Geometry: final body of the model. Coordinates: model frame, mm. A direction names the side the tool comes from. Round coordinates to 2 decimals unless told otherwise and drop trailing zeros. Loops run counter-clockwise (first coordinate to the right, second up) from the corner with the lowest first, then second, coordinate; pieces in that order, holes last. Notation, with made-up numbers: M -31,69 L 27,69 A25 ccw 27,91 Z; hole C -8,42 d9. An arc over 180 degrees is marked long. Return JSON: item names as keys, results as strings.
from build123d import *

# Parameters (mm, degrees)
BOSS_EXTRUDE2_DEPTH      = 100
SKETCH4_W                = 245
SKETCH4_H                = 170
CUT_EXTRUDE2_DEPTH       = 70
CUT_EXTRUDE12_DEPTH      = 434.077648927
CUT_EXTRUDE12_DEPTH_BACK = 434.077648927
CUT_EXTRUDE13_DEPTH      = 122.5
CUT_EXTRUDE14_DEPTH      = 122.5
SKETCH16_W               = 43.138722299
SKETCH16_H               = 40.379444726
CUT_EXTRUDE15_DEPTH      = 30
SKETCH17_W               = 15
SKETCH17_H               = 16
SKETCH17_W_2             = 18.622276722
SKETCH17_H_2             = 25.273514742
CUT_EXTRUDE16_DEPTH      = 10
BOSS_EXTRUDE3_DEPTH      = 25
SKETCH19_W               = 25
SKETCH19_H               = 20
CUT_EXTRUDE17_DEPTH      = 15


with BuildPart() as part:
    # Sketch1 → Boss-Extrude2 (new body)
    with BuildSketch(Plane(origin=(0, 0, 0), x_dir=(1, 0, 0), z_dir=(0, 1, 0))):
        with BuildLine():
            Line((0, -10), (0, -390))
            ThreePointArc((0, -390), (2.928932188, -397.071067812), (10, -400))
            Line((10, -400), (255, -400))
            ThreePointArc((255, -400), (262.071067812, -397.071067812), (265, -390))
            Line((265, -390), (265, -10))
            ThreePointArc((265, -10), (262.071067812, -2.928932188), (255, 0))
            Line((255, 0), (10, 0))
            ThreePointArc((10, 0), (2.928932188, -2.928932188), (0, -10))
        make_face()
    extrude(amount=BOSS_EXTRUDE2_DEPTH)

    # Sketch4 → Cut-Extrude2 (cut)
    with BuildSketch(Plane(origin=(0, 100, 0), x_dir=(1, 0, 0), z_dir=(0, 1, 0))):
        with Locations((132.5, -265)):
            Rectangle(SKETCH4_W, SKETCH4_H)
    extrude(amount=-CUT_EXTRUDE2_DEPTH, mode=Mode.SUBTRACT)

    # Sketch10 → Cut-Extrude12 (cut, two sides: drawn at the far end of the back side and taken through both)
    with BuildSketch(Plane(origin=(132.5, 0, 0), x_dir=(0, 0, -1), z_dir=(1, 0, 0)).offset(-CUT_EXTRUDE12_DEPTH_BACK)):
        Polygon((-400, 60), (-370, 100), (-400, 100), align=None)
    extrude(amount=CUT_EXTRUDE12_DEPTH + CUT_EXTRUDE12_DEPTH_BACK, mode=Mode.SUBTRACT)

    # Sketch14 → Cut-Extrude13 (cut, symmetric)
    with BuildSketch(Plane(origin=(132.5, 0, 0), x_dir=(0, 0, -1), z_dir=(1, 0, 0))):
        Polygon((-390, 10), (-360, 10), (-360, 96), (-368, 96), (-390, 66.666666667), align=None)
    extrude(amount=CUT_EXTRUDE13_DEPTH, both=True, mode=Mode.SUBTRACT)

    # Sketch15 → Cut-Extrude14 (cut, symmetric)
    with BuildSketch(Plane(origin=(132.5, 0, 0), x_dir=(0, 0, -1), z_dir=(1, 0, 0))):
        Polygon((-360, 9.784104138), (-360, 20), (-170, 20), (-170, 95), (-15, 95), (-15, 10), align=None)
    extrude(amount=CUT_EXTRUDE14_DEPTH, both=True, mode=Mode.SUBTRACT)

    # Sketch16 → Cut-Extrude15 (cut)
    with BuildSketch(Plane(origin=(0, 0, 0), x_dir=(-1, 0, 0), z_dir=(0, 0, -1))):
        with BuildLine():
            Line((-240.140690251, 79.23821095), (-190.467776295, 79.23821095))
            ThreePointArc((-190.467776295, 79.23821095), (-188.532467959, 77.302902614), (-190.467776295, 75.367594278))
            Line((-190.467776295, 75.367594278), (-240.140690251, 75.367594278))
            ThreePointArc((-240.140690251, 75.367594278), (-242.075998587, 77.302902614), (-240.140690251, 79.23821095))
        make_face()
        with BuildLine():
            Line((-183.801714249, 79.23821095), (-136.494177148, 79.23821095))
            ThreePointArc((-136.494177148, 79.23821095), (-134.558868812, 77.302902614), (-136.494177148, 75.367594278))
            Line((-136.494177148, 75.367594278), (-183.801714249, 75.367594278))
            ThreePointArc((-183.801714249, 75.367594278), (-185.737022585, 77.302902614), (-183.801714249, 79.23821095))
        make_face()
        with BuildLine():
            Line((-239.932606186, 72.357114645), (-190.25969223, 72.357114645))
            ThreePointArc((-190.25969223, 72.357114645), (-188.324383894, 70.421806309), (-190.25969223, 68.486497973))
            Line((-190.25969223, 68.486497973), (-239.932606186, 68.486497973))
            ThreePointArc((-239.932606186, 68.486497973), (-241.867914521, 70.421806309), (-239.932606186, 72.357114645))
        make_face()
        with BuildLine():
            Line((-183.593630184, 72.357114645), (-136.286093083, 72.357114645))
            ThreePointArc((-136.286093083, 72.357114645), (-134.350784747, 70.421806309), (-136.286093083, 68.486497973))
            Line((-136.286093083, 68.486497973), (-183.593630184, 68.486497973))
            ThreePointArc((-183.593630184, 68.486497973), (-185.52893852, 70.421806309), (-183.593630184, 72.357114645))
        make_face()
        with BuildLine():
            Line((-239.825089056, 65.476018339), (-190.1521751, 65.476018339))
            ThreePointArc((-190.1521751, 65.476018339), (-188.216866764, 63.540710003), (-190.1521751, 61.605401667))
            Line((-190.1521751, 61.605401667), (-239.825089056, 61.605401667))
            ThreePointArc((-239.825089056, 61.605401667), (-241.760397392, 63.540710003), (-239.825089056, 65.476018339))
        make_face()
        with BuildLine():
            Line((-183.486113054, 65.476018339), (-136.178575953, 65.476018339))
            ThreePointArc((-136.178575953, 65.476018339), (-134.243267617, 63.540710003), (-136.178575953, 61.605401667))
            Line((-136.178575953, 61.605401667), (-183.486113054, 61.605401667))
            ThreePointArc((-183.486113054, 61.605401667), (-185.42142139, 63.540710003), (-183.486113054, 65.476018339))
        make_face()
        with BuildLine():
            Line((-239.617004991, 58.594922033), (-189.944091035, 58.594922033))
            ThreePointArc((-189.944091035, 58.594922033), (-188.008782699, 56.659613697), (-189.944091035, 54.724305362))
            Line((-189.944091035, 54.724305362), (-239.617004991, 54.724305362))
            ThreePointArc((-239.617004991, 54.724305362), (-241.552313326, 56.659613697), (-239.617004991, 58.594922033))
        make_face()
        with BuildLine():
            Line((-183.278028989, 58.594922033), (-135.970491888, 58.594922033))
            ThreePointArc((-135.970491888, 58.594922033), (-134.035183552, 56.659613697), (-135.970491888, 54.724305362))
            Line((-135.970491888, 54.724305362), (-183.278028989, 54.724305362))
            ThreePointArc((-183.278028989, 54.724305362), (-185.213337325, 56.659613697), (-183.278028989, 58.594922033))
        make_face()
        with BuildLine():
            Line((-239.918705797, 44.187626644), (-190.245791841, 44.187626644))
            ThreePointArc((-190.245791841, 44.187626644), (-188.310483505, 42.252318308), (-190.245791841, 40.317009972))
            Line((-190.245791841, 40.317009972), (-239.918705797, 40.317009972))
            ThreePointArc((-239.918705797, 40.317009972), (-241.854014133, 42.252318308), (-239.918705797, 44.187626644))
        make_face()
        with BuildLine():
            Line((-183.579729795, 44.187626644), (-136.272192694, 44.187626644))
            ThreePointArc((-136.272192694, 44.187626644), (-134.336884358, 42.252318308), (-136.272192694, 40.317009972))
            Line((-136.272192694, 40.317009972), (-183.579729795, 40.317009972))
            ThreePointArc((-183.579729795, 40.317009972), (-185.515038131, 42.252318308), (-183.579729795, 44.187626644))
        make_face()
        with BuildLine():
            Line((-239.710621732, 37.306530338), (-190.037707776, 37.306530338))
            ThreePointArc((-190.037707776, 37.306530338), (-188.10239944, 35.371222002), (-190.037707776, 33.435913666))
            Line((-190.037707776, 33.435913666), (-239.710621732, 33.435913666))
            ThreePointArc((-239.710621732, 33.435913666), (-241.645930068, 35.371222002), (-239.710621732, 37.306530338))
        make_face()
        with BuildLine():
            Line((-183.37164573, 37.306530338), (-136.064108629, 37.306530338))
            ThreePointArc((-136.064108629, 37.306530338), (-134.128800293, 35.371222002), (-136.064108629, 33.435913666))
            Line((-136.064108629, 33.435913666), (-183.37164573, 33.435913666))
            ThreePointArc((-183.37164573, 33.435913666), (-185.306954066, 35.371222002), (-183.37164573, 37.306530338))
        make_face()
        with BuildLine():
            Line((-239.603104602, 30.425434033), (-189.930190646, 30.425434033))
            ThreePointArc((-189.930190646, 30.425434033), (-187.99488231, 28.490125697), (-189.930190646, 26.554817361))
            Line((-189.930190646, 26.554817361), (-239.603104602, 26.554817361))
            ThreePointArc((-239.603104602, 26.554817361), (-241.538412938, 28.490125697), (-239.603104602, 30.425434033))
        make_face()
        with BuildLine():
            Line((-183.2641286, 30.425434033), (-135.956591499, 30.425434033))
            ThreePointArc((-135.956591499, 30.425434033), (-134.021283163, 28.490125697), (-135.956591499, 26.554817361))
            Line((-135.956591499, 26.554817361), (-183.2641286, 26.554817361))
            ThreePointArc((-183.2641286, 26.554817361), (-185.199436936, 28.490125697), (-183.2641286, 30.425434033))
        make_face()
        with BuildLine():
            Line((-239.395020537, 23.544337727), (-189.722106581, 23.544337727))
            ThreePointArc((-189.722106581, 23.544337727), (-187.786798245, 21.609029391), (-189.722106581, 19.673721055))
            Line((-189.722106581, 19.673721055), (-239.395020537, 19.673721055))
            ThreePointArc((-239.395020537, 19.673721055), (-241.330328873, 21.609029391), (-239.395020537, 23.544337727))
        make_face()
        with BuildLine():
            Line((-183.056044535, 23.544337727), (-135.748507434, 23.544337727))
            ThreePointArc((-135.748507434, 23.544337727), (-133.813199098, 21.609029391), (-135.748507434, 19.673721055))
            Line((-135.748507434, 19.673721055), (-183.056044535, 19.673721055))
            ThreePointArc((-183.056044535, 19.673721055), (-184.991352871, 21.609029391), (-183.056044535, 23.544337727))
        make_face()
        with Locations((-62.397436661, 30.189722363)):
            Rectangle(SKETCH16_W, SKETCH16_H)
    extrude(amount=-CUT_EXTRUDE15_DEPTH, mode=Mode.SUBTRACT)

    # Sketch17 → Cut-Extrude16 (cut)
    with BuildSketch(Plane(origin=(0, 213.6, 284.8), x_dir=(1, 0, 0), z_dir=(0, 0.5999999999999998, 0.8000000000000004))):
        with Locations((68, -165)):
            Rectangle(SKETCH17_W, SKETCH17_H)
        with Locations((197, -165)):
            Rectangle(SKETCH17_W, SKETCH17_H)
        with Locations((132.148099668, -169.636757371)):
            Rectangle(SKETCH17_W_2, SKETCH17_H_2)
    extrude(amount=-CUT_EXTRUDE16_DEPTH, mode=Mode.SUBTRACT)

    # Sketch18 → Boss-Extrude3 (add)
    with BuildSketch(Plane(origin=(0, 30, 0), x_dir=(1, 0, 0), z_dir=(0, 1, 0))):
        with BuildLine():
            Line((10, -180), (10, -204.729927007))
            Line((10, -204.729927007), (30, -204.729927007))
            ThreePointArc((30, -204.729927007), (33.43872324, -203.359690427), (34.99270073, -200))
            Line((34.99270073, -200), (34.99270073, -180))
            Line((34.99270073, -180), (10, -180))
        make_face()
        with BuildLine():
            Line((255, -350), (255, -324.14910859))
            Line((255, -324.14910859), (235, -324.14910859))
            ThreePointArc((235, -324.14910859), (231.175444009, -325.928429861), (230.072933549, -330))
            Line((230.072933549, -330), (230.072933549, -350))
            Line((230.072933549, -350), (255, -350))
        make_face()
    extrude(amount=BOSS_EXTRUDE3_DEPTH)

    # Sketch19 → Cut-Extrude17 (cut)
    with BuildSketch(Plane.XY.offset(180)):
        with Locations((67.49270073, 42.5)):
            Rectangle(SKETCH19_W, SKETCH19_H)
    extrude(amount=-CUT_EXTRUDE17_DEPTH, mode=Mode.SUBTRACT)


solid = part.part
Q1. Section query D-D (z = 161.5). Output: boundary loops of the cut face in (x, y).
Determined:
{"outline": "M 0,0 L 265,0 L 265,100 L 0,100 Z; hole M 10,9.91 L 255,9.91 L 255,95 L 10,95 Z"}
Q2. Section query A-A (x = 69). State how many separate pieces and enclosed holes the cut face has, plus the area to 3 significant figures.
Determined:
{"separate pieces": "3", "enclosed holes": "0", "area": "9,260 mm^2"}
Q3. Section query B-B (z = 299). Output: boundary loops of the cut face in (x, y), plus the area to 3 significant figures.
Determined:
{"outline": "M 0,0 L 265,0 L 265,100 L 255,100 L 255,30 L 10,30 L 10,100 L 0,100 Z; hole M 10,9.82 L 255,9.82 L 255,20 L 10,20 Z", "area": "6,860 mm^2"}
Q4. Reachability of faces 4 (the flat face through (134, 96, 364)), 5 (the flat face through (230.073, 42, 340)), 6 (the flat face through (215, 44.188, 7)), 7 (the flat face through (134, 49, 0)), 8 (the cylindrical face through (261.99, 36.15, 397.15)) from +Z, -Z, +X, -X, +Y, -Y: full face, straight path, thin tool, end or side. Return the list, or none.
Determined:
{"face 4": "none", "face 5": "+Y", "face 6": "-Z", "face 7": "-Z, +X, -X, +Y, -Y", "face 8": "+Z, +X, +Y, -Y"}
Q5. Pull-direction query (X, two-part tool) for faces 1 (the cylindrical face through (262.15, 49.3, 3.01)), 2 (the cylindrical face through (3.01, 49.3, 2.85)), 3 (the flat face through (255, 53, 163)); classes: pulls with the +X half, pulls with the -X half, needs draft (parallel to the pull), parting line crosses it, or undercut.
Determined:
{"face 1": "pulls with the +X half", "face 2": "pulls with the -X half", "face 3": "undercut"}
Q6. Pin query (flat end, axial travel): pin 1 (1 mm diameter, centred on x = 106.5, z = 338.5, fed in from +Y); pin 2 (12.5 mm diameter, centred on x = 22.5, z = 187, fed in from +Y). Return the tip coordinate at first contact, or that it passes through.
Determined:
{"pin 1": "stops at y = 30", "pin 2": "stops at y = 55"}
Q7. Material intervals for L1, parallel to Z at x = 23.5, y = 21.5; L2, parallel to Z at x = 224.5, y = 45; L3, parallel to Z at x = 138.5, y = 73, sorted ascending.
Determined:
{"L1": "z = 0 to 15, 170 to 360, 390 to 400", "L2": "z = 0 to 15, 170 to 180, 350 to 360, 390 to 400", "L3": "z = 0 to 15, 170 to 180, 350 to 360"}
